Part print with two shaded views. Sizes in mm from the minimum x, y, z corner. Coordinates: 2 decimals unless noted, no trailing zeros. Loops run counter-clockwise (first coordinate to the right, second up) from the corner with the lowest first, then second, coordinate; pieces in that order, holes last.
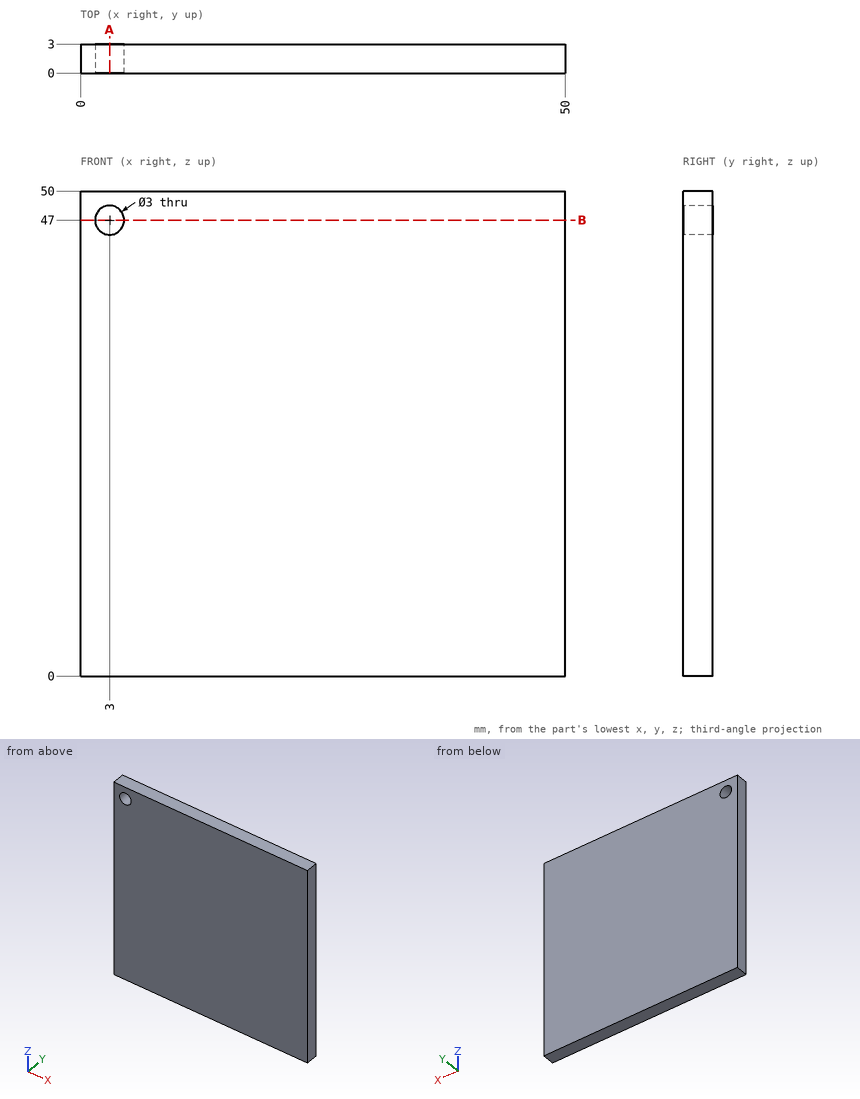
Q1. Slice it at B-B (z = 47). List the corners of the cut face in (x, y), and give its area (3 significant figures).
Answers:
outline: (0, 0) - (1.5, 0) - (1.5, 3) - (0, 3) - close; (4.5, 0) - (50, 0) - (50, 3) - (4.5, 3) - close
area: 141 mm2
Q2. Slice it at A-A (x = 3). List the corners of the cut face in (y, z), and give its area (3 significant figures).
Answers:
outline: (0, 0) - (3, 0) - (3, 45.5) - (0, 45.5) - close; (0, 48.5) - (3, 48.5) - (3, 50) - (0, 50) - close
area: 141 mm2
Q3. Drill centre lines: line 1 (Z direction, x = 3, y = 1.4); line 2 (X direction, y = 1.75, z = 46). Where is each one in solid material? Low to high.
Answers:
line 1: z = 0 to 45.5, 48.5 to 50
line 2: x = 0 to 1.88, 4.12 to 50
